Check sheet for the modelled part. Datum: model origin and axes. Units: mm. Round coordinates to 2 decimals unless told otherwise and drop trailing zeros. Loops run counter-clockwise (first coordinate to the right, second up) from the corner with the lowest first, then second, coordinate; pieces in that order, holes last. Notation, with made-up numbers: (19, -5) -> (39, -5) arc R26 cw to (39, 13) -> close; hole circle Ø2 at (-24, 18.25). An arc over 180 degrees is marked (long way). Use one line per item in the form item = value. Start each with the question number.
(1) Draft check along Z on faces 1 (the flat face through (-22.35, -8, 0)), 2 (the flat face through (0, -8, -13)), 3 (the flat face through (22.35, -8, 0)), 4 (the flat face through (0, -8, 13)). Enter one of: released by +Z, released by -Z, zero draft, split by the parting line, or undercut.
(2) Sectioned sample at A-A (y = -1.5). Record the cut outline in (x, z), and give its area (3 significant figures).
(3) Material ranges on probe 1 along X at (y, z) = (-4.25, -9); probe 2 along Y at (x, z) = (22.5, -4.25), recorded low to high. Write a range as [from, to].
(4) Sectioned sample at B-B (y = -6). Record the cut outline in (x, z), and give its area (3 significant figures).
from build123d import *

# Parameters (mm, degrees)
F0_W     = 44.7
F0_H     = 26
F1_DEPTH = 16.9
F3_DEPTH = 4


with BuildPart() as f1:
    # F0 (on Front) → F1 (new body)
    with BuildSketch(Plane.XZ):
        Rectangle(F0_W, F0_H)
    extrude(amount=F1_DEPTH)

    # F2 (on face) → F3 (join)
    with BuildSketch(Plane.YZ.offset(22.35)):
        with BuildLine():
            ThreePointArc((-8.45, -3.325), (-11.625, -6.5), (-8.45, -9.675))
            Line((-8.45, -9.675), (-8.45, -3.325))
        make_face()
        with BuildLine():
            Line((-8.45, -3.325), (-8.45, -9.675))
            ThreePointArc((-8.45, -9.675), (-6.2049359697, -8.7450640303), (-5.275, -6.5))
            ThreePointArc((-5.275, -6.5), (-6.2049359697, -4.2549359697), (-8.45, -3.325))
        make_face()
        with BuildLine():
            ThreePointArc((-8.45, 9.675), (-11.625, 6.5), (-8.45, 3.325))
            Line((-8.45, 3.325), (-8.45, 6.5))
            Line((-8.45, 6.5), (-8.45, 9.675))
        make_face()
        with BuildLine():
            Line((-8.45, 6.5), (-8.45, 3.325))
            ThreePointArc((-8.45, 3.325), (-6.2049359697, 4.2549359697), (-5.275, 6.5))
            ThreePointArc((-5.275, 6.5), (-6.2049359697, 8.7450640303), (-8.45, 9.675))
            Line((-8.45, 9.675), (-8.45, 6.5))
        make_face()
    extrude(amount=F3_DEPTH)


solid = f1.part
Checks:
q1.face_1 = zero draft
q1.face_2 = released by -Z
q1.face_3 = undercut
q1.face_4 = released by +Z
q2.outline = (-22.35, -13) -> (22.35, -13) -> (22.35, 13) -> (-22.35, 13) -> close
q2.area = 1,160 mm2
q3.probe_1 = [-22.35, 22.35]
q3.probe_2 = [-10.69, -6.21]
q4.outline = (-22.35, -13) -> (22.35, -13) -> (22.35, -8.52) -> (26.35, -8.52) -> (26.35, -4.48) -> (22.35, -4.48) -> (22.35, 4.48) -> (26.35, 4.48) -> (26.35, 8.52) -> (22.35, 8.52) -> (22.35, 13) -> (-22.35, 13) -> close
q4.area = 1,190 mm2
